from build123d import *

# Parameters (mm, degrees)
SKETCH1_W           = 23.4
SKETCH1_H           = 29
SKETCH1_R           = 1
BOSS_EXTRUDE1_DEPTH = 3
FILLET1_R           = 2
SKETCH8_R           = 1
CUT_EXTRUDE5_DEPTH  = 10
SKETCH10_R          = 1.95
CUT_EXTRUDE6_DEPTH  = 10
SKETCH11_R          = 1.8
CUT_EXTRUDE7_DEPTH  = 1.45


with BuildPart() as part:
    # Sketch1 → Boss-Extrude1 (new body)
    with BuildSketch(Plane(origin=(0, 0, 0), x_dir=(1, 0, 0), z_dir=(0, 1, 0))):
        Rectangle(SKETCH1_W, SKETCH1_H)
        with Locations((9, 9.3)):
            Circle(SKETCH1_R, mode=Mode.SUBTRACT)
        with Locations((9, -8.5)):
            Circle(SKETCH1_R, mode=Mode.SUBTRACT)
        with Locations((-9, -8.5)):
            Circle(SKETCH1_R, mode=Mode.SUBTRACT)
        with Locations((1.7, -8.5)):
            Circle(SKETCH1_R, mode=Mode.SUBTRACT)
    extrude(amount=BOSS_EXTRUDE1_DEPTH)

    # Fillet1
    fillet1_edges = [part.edges().sort_by_distance(p)[0] for p in [
        (11.7, 1.5, 14.5),
        (-11.7, 1.5, 14.5),
        (-11.7, 1.5, -14.5),
        (11.7, 1.5, -14.5),
    ]]
    fillet(fillet1_edges, radius=FILLET1_R)

    # Sketch8 → Cut-Extrude5 (cut)
    with BuildSketch(Plane(origin=(0, 3, 0), x_dir=(1, 0, 0), z_dir=(0, 1, 0))):
        with Locations((1.7, 9.3)):
            Circle(SKETCH8_R)
        with Locations((-9, 9.3)):
            Circle(SKETCH8_R)
    extrude(amount=-CUT_EXTRUDE5_DEPTH, mode=Mode.SUBTRACT)

    # Sketch10 → Cut-Extrude6 (cut)
    with BuildSketch(Plane(origin=(0, 3, 0), x_dir=(1, 0, 0), z_dir=(0, 1, 0))):
        with Locations((-2.328177417, 0.5)):
            Circle(SKETCH10_R)
    extrude(amount=-CUT_EXTRUDE6_DEPTH, mode=Mode.SUBTRACT)

    # Sketch11 → Cut-Extrude7 (cut)
    with BuildSketch(Plane(origin=(0, 3, 0), x_dir=(1, 0, 0), z_dir=(0, 1, 0))):
        with Locations((-9, -8.5)):
            Circle(SKETCH11_R)
        with Locations((1.671822583, -9)):
            Circle(SKETCH11_R)
        with Locations((9, -8.5)):
            Circle(SKETCH11_R)
        with Locations((9, 9.3)):
            Circle(SKETCH11_R)
        with Locations((1.7, 9.3)):
            Circle(SKETCH11_R)
        with Locations((-9, 9.3)):
            Circle(SKETCH11_R)
    extrude(amount=-CUT_EXTRUDE7_DEPTH, mode=Mode.SUBTRACT)


solid = part.part
The listing builds one solid part. Answer for the finished solid, in the listing's coordinates (mm). A direction names the side the tool comes from. Coordinates: 2 decimals unless noted, no trailing zeros. Order: outer loops, then holes, each group sorted by start corner. A loop starts at its lowest first (then second) coordinate and runs counter-clockwise, first axis right, second up.
Q1. Given P1, Ø1.8, axis at x = -8.5, z = 8.5, coming from the +Y side, flat-ended and moving along its own axis, determine where the tip first touches the part or whether it passes through.
Q2. A cutting plane is placed at C-C, the plane x = -9. Write down the section's boundary in (y, z).
Q3. A cutting plane is placed at D-D, the plane x = -1.25. Write down the section's boundary in (y, z).
Q4. Consider line 1 (Z direction, x = 9, y = 0.6); line 2 (Z direction, x = -9, y = 2.6); line 3 (X direction, y = 0.9, z = -0.5). Determine where each line is inside the solid, lowest interval first.
Q5. Which of the six approach directions +Z, -Z, +X, -X, +Y, -Y give full straight-line access (tool end or side, diameter ignored) to faces 5 (the face through (2, 1.55, 10)), 6 (the face through (11.1, 1.52, -13.93))?
Q6. A cutting plane is placed at B-B, the plane y = 0.6. Write down the section's boundary in (x, z), and give its area (3 significant figures).
Q7. For a pull along X with two mould halves and no side action, classify faces 1 (the face through (8.87, 0.76, 7.51)), 2 (the face through (-11.13, 1.52, -13.9)), 3 (the face through (1.57, 0.76, 7.51)), 4 (the face through (0, 1, -14.5)) as pulls with the +X half, pulls with the -X half, needs draft (parallel to the pull), parting line crosses it, or undercut.
Q8. A cutting plane is placed at A-A, the plane z = -9.3. Write down the section's boundary in (x, y), and give its area (3 significant figures).
Answers follow:
1. P1: stops at y = 1.55
2. outline: (0, -14.5) - (3, -14.5) - (3, -11.1) - (1.55, -11.1) - (1.55, -10.3) - (0, -10.3) - close; (0, -8.3) - (1.55, -8.3) - (1.55, -7.5) - (3, -7.5) - (3, 6.7) - (1.55, 6.7) - (1.55, 7.5) - (0, 7.5) - close; (0, 9.5) - (1.55, 9.5) - (1.55, 10.3) - (3, 10.3) - (3, 14.5) - (0, 14.5) - close
3. outline: (0, -14.5) - (3, -14.5) - (3, -2.12) - (0, -2.12) - close; (0, 1.12) - (3, 1.12) - (3, 14.5) - (0, 14.5) - close
4. line 1: z = -14.5 to -10.3, -8.3 to 7.5, 9.5 to 14.5
4. line 2: z = -14.5 to -11.1, -7.5 to 6.7, 10.3 to 14.5
4. line 3: x = -11.7 to -4.28, -0.38 to 11.7
5. face 5: +Y
5. face 6: -Z, +X, +Y, -Y
6. outline: (-11.7, -12.5) arc R2 ccw to (-9.7, -14.5) - (9.7, -14.5) arc R2 ccw to (11.7, -12.5) - (11.7, 12.5) arc R2 ccw to (9.7, 14.5) - (-9.7, 14.5) arc R2 ccw to (-11.7, 12.5) - close; hole circle Ø2 at (-9, -9.3); hole circle Ø2 at (-9, 8.5); hole circle Ø3.9 at (-2.33, -0.5); hole circle Ø2 at (1.7, -9.3); hole circle Ø2 at (1.7, 8.5); hole circle Ø2 at (9, -9.3); hole circle Ø2 at (9, 8.5)
6. area: 644 mm2
7. face 1: undercut
7. face 2: pulls with the -X half
7. face 3: undercut
7. face 4: needs draft
8. outline: (-11.7, 0) - (-10, 0) - (-10, 1.55) - (-10.8, 1.55) - (-10.8, 3) - (-11.7, 3) - close; (-8, 0) - (0.7, 0) - (0.7, 1.55) - (-0.1, 1.55) - (-0.1, 3) - (-7.2, 3) - (-7.2, 1.55) - (-8, 1.55) - close; (2.7, 0) - (8, 0) - (8, 1.55) - (7.2, 1.55) - (7.2, 3) - (3.5, 3) - (3.5, 1.55) - (2.7, 1.55) - close; (10, 0) - (11.7, 0) - (11.7, 3) - (10.8, 3) - (10.8, 1.55) - (10, 1.55) - close
8. area: 45.2 mm2
